Design review of the part built by this model. Coordinates are the model's own, in mm. A direction names the side the tool comes from. Round coordinates to 2 decimals unless told otherwise and drop trailing zeros. Loops run counter-clockwise (first coordinate to the right, second up) from the corner with the lowest first, then second, coordinate; pieces in that order, holes last. Notation, with made-up numbers: (55.5, 78) - (90.5, 78) arc R21 ccw to (90.5, 97) - close; hole circle Ø5 at (73.25, 19.25). An arc over 180 degrees is marked (long way). Use one line per item in the form item = value. Start each with the question number.
(1) We need section C-C, the plane z = 2.25. Write out the cut boundary in (x, y), then the cut area to 3 significant figures.
(2) Machinability: for faces 5 (the flat face through (727.339, 342, 3)), 6 (the flat face through (736, 347.006, 3)), 7 (the flat face through (740.339, 348, 3)), which of the approach directions +Z, -Z, +X, -X, +Y, -Y give a long, thin tool a straight path to every point of the face, cutting with its end or side? Answer none if there is none.
(3) Wall thickness on probe 1 along Y at (x, z) = (738.5, 5.1); probe 2 along Y at (x, z) = (732, 1.9); probe 3 along X at (y, z) = (343, 4.65): over which ranges is each line inside the solid? List them lowest first. Write a range as [from, to].
(4) For pin 1 (1.4 mm diameter, centred on y = 344, z = 4, fed in from -X); pin 2 (4 mm diameter, centred on x = 741, y = 346, fed in from +Z); pin 3 (1.3 mm diameter, centred on y = 345, z = 2, fed in from -X), all flat-tipped, find the tip position at first contact; note any pin that passes through.
(5) We need section D-D, the plane y = 345. Write out the cut boundary in (x, z), then the cut area to 3 significant figures.
(6) We need section A-A, the plane x = 735.25. Write out the cut boundary in (y, z), then the cut area to 3 significant figures.
(7) We need section B-B, the plane y = 343.5. Write out the cut boundary in (x, z).
(8) The part is to be moulded in two halves that separate along X. For faces 1 (the flat face through (737.939, 348, 3)), 2 (the flat face through (741, 348, 5.64)), 3 (the cylindrical face through (748.63, 341.31, 2.86)), 4 (the flat face through (740.339, 344, 3)), say which applies: released by +X, released by -X, zero draft, split by the parting line, or undercut.
from build123d import *

# Parameters (mm, degrees)
BOSS_EXTRUDE2_DEPTH = 5.64
FILLET1_R           = 2.5


with BuildPart() as part:
    # Sketch1 → Boss-Extrude2 (new body)
    with BuildSketch(Plane.XY):
        Polygon((727.33944815, 350.756300382), (749.33944815, 350.756300382), (749.33944815, 340.556300382), (727.33944815, 340.556300382), (727.33944815, 342.556300382), (733.33944815, 342.556300382), (733.33944815, 344.306300382), (737.93944815, 344.306300382), (737.93944815, 342.866300382), (740.33944815, 342.866300382), (740.33944815, 344.306300382), (742.33944815, 344.306300382), (742.33944815, 347.006300382), (740.33944815, 347.006300382), (740.33944815, 348.446300382), (737.93944815, 348.446300382), (737.93944815, 347.006300382), (733.33944815, 347.006300382), (733.33944815, 348.756300382), (727.33944815, 348.756300382), align=None)
    extrude(amount=BOSS_EXTRUDE2_DEPTH)

    # Fillet1
    fillet1_edges = [part.edges().sort_by_distance(p)[0] for p in [
        (749.33944815, 350.756300382, 2.82),
        (749.33944815, 340.556300382, 2.82),
    ]]
    fillet(fillet1_edges, radius=FILLET1_R)


solid = part.part
Data:
q1.outline = (727.34, 340.56) - (746.84, 340.56) arc R2.5 ccw to (749.34, 343.06) - (749.34, 348.26) arc R2.5 ccw to (746.84, 350.76) - (727.34, 350.76) - (727.34, 348.76) - (733.34, 348.76) - (733.34, 347.01) - (737.94, 347.01) - (737.94, 348.45) - (740.34, 348.45) - (740.34, 347.01) - (742.34, 347.01) - (742.34, 344.31) - (740.34, 344.31) - (740.34, 342.87) - (737.94, 342.87) - (737.94, 344.31) - (733.34, 344.31) - (733.34, 342.56) - (727.34, 342.56) - close
q1.area = 153 mm^2
q2.face_5 = +Z, -Z, -X, +Y, -Y
q2.face_6 = +Z, -Z, -X
q2.face_7 = +Z, -Z
q3.probe_1 = [340.56, 342.87], [348.45, 350.76]
q3.probe_2 = [340.56, 342.56], [348.76, 350.76]
q3.probe_3 = [733.34, 737.94], [740.34, 749.34]
q4.pin_1 = 733.34
q4.pin_2 = 5.64
q4.pin_3 = 742.34
q5.outline = (742.34, 0) - (749.34, 0) - (749.34, 5.64) - (742.34, 5.64) - close
q5.area = 39.5 mm^2
q6.outline = (340.56, 0) - (344.31, 0) - (344.31, 5.64) - (340.56, 5.64) - close; (347.01, 0) - (350.76, 0) - (350.76, 5.64) - (347.01, 5.64) - close
q6.area = 42.3 mm^2
q7.outline = (733.34, 0) - (737.94, 0) - (737.94, 5.64) - (733.34, 5.64) - close; (740.34, 0) - (749.34, 0) - (749.34, 5.64) - (740.34, 5.64) - close
q8.face_1 = undercut
q8.face_2 = zero draft
q8.face_3 = released by +X
q8.face_4 = undercut
